Source: three-view drawing plus pictorial views. Frame: mm from the lowest corner of the part. A direction names the side the tool comes from. Give positions to 0.01 mm unless a question says otherwise; leave off trailing zeros. Order: outer loops, then holes, each group sorted by start corner. A loop starts at its lowest first (then second) coordinate and runs counter-clockwise, first axis right, second up.
1) Section C-C, the plane z = 1.55. Return loops of the section in (x, y).
2) Section B-B, the plane y = 17.25. Return loops of the section in (x, z).
3) First-contact query: P1, Ø0.5, axis at y = 13, z = 2, coming from the -X side; P2, Ø1.4, axis at y = 8.5, z = 2, coming from the +X side; P3, Ø0.5, axis at x = 6, z = 2, coming from the -Y side. Flat tips, straight axial feed; report the tip coordinate or a pass-through.
4) Access query for the marked faces 1, 2, 3 and 4. Directions: +Z, -Z, +X, -X, +Y, -Y. A direction counts if a zero-diameter tool reaches every point of the face in a straight line with its end or side. Return the directions, or none.
5) Section A-A, the plane x = 8. Return loops of the section in (y, z), plus the area to 3 significant figures.
6) Draft query along X for the marked faces 5, 6, 7 and 8. Return one class per face: released by +X, released by -X, zero draft, split by the parting line, or undercut.
7) Section D-D, the plane x = 4. Return loops of the section in (y, z), plus the area to 3 significant figures.
8) Material intervals for line 1 (X direction, y = 8, z = 0.65); line 2 (X direction, y = 9, z = 1.4); line 3 (Z direction, x = 1, y = 9.5), sorted ascending.
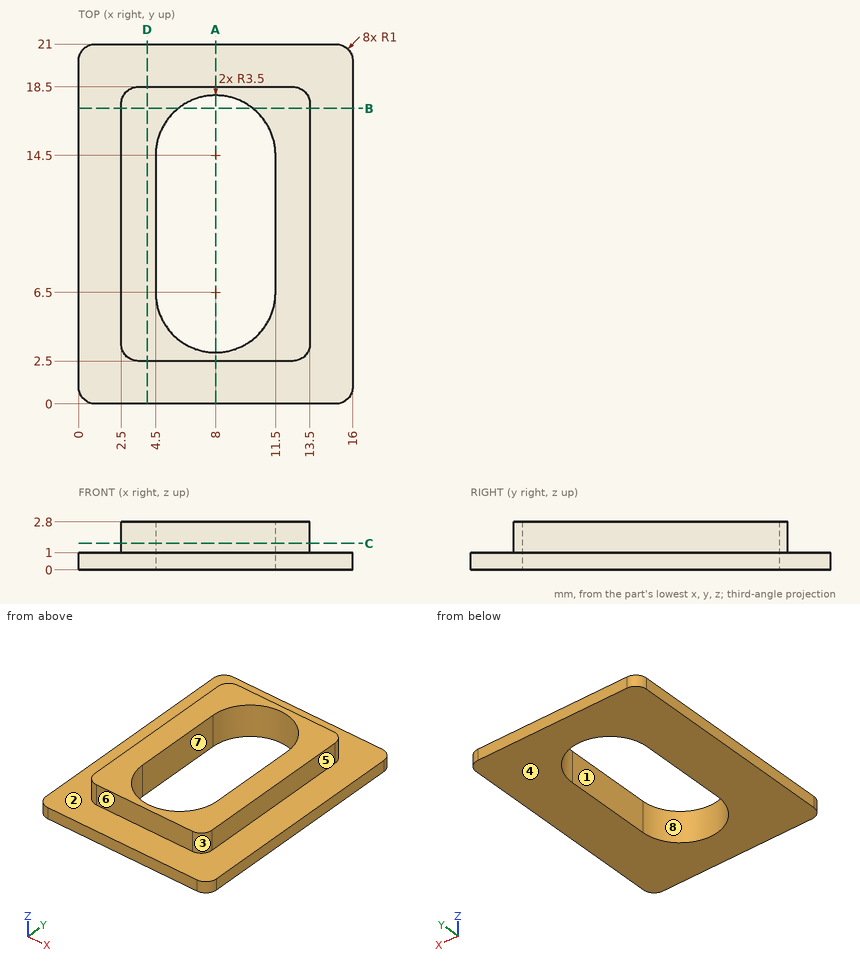
From the geometry:
1. outline: (2.5, 3.5) arc R1 ccw to (3.5, 2.5) - (12.5, 2.5) arc R1 ccw to (13.5, 3.5) - (13.5, 17.5) arc R1 ccw to (12.5, 18.5) - (3.5, 18.5) arc R1 ccw to (2.5, 17.5) - close; hole (4.5, 6.5) arc R3.5 ccw to (11.5, 6.5) - (11.5, 14.5) arc R3.5 ccw to (4.5, 14.5) - close
2. outline: (0, 0) - (5.83, 0) - (5.83, 2.8) - (2.5, 2.8) - (2.5, 1) - (0, 1) - close; (10.17, 0) - (16, 0) - (16, 1) - (13.5, 1) - (13.5, 2.8) - (10.17, 2.8) - close
3. P1: stops at x = 2.5
3. P2: stops at x = 13.5
3. P3: stops at y = 2.5
4. face 1: +Z, -Z
4. face 2: +Z
4. face 3: +Z, +X, -Y
4. face 4: -Z, +X, -X, +Y, -Y
5. outline: (0, 0) - (3, 0) - (3, 2.8) - (2.5, 2.8) - (2.5, 1) - (0, 1) - close; (18, 0) - (21, 0) - (21, 1) - (18.5, 1) - (18.5, 2.8) - (18, 2.8) - close
5. area: 7.80 mm2
6. face 5: released by +X
6. face 6: zero draft
6. face 7: undercut
6. face 8: undercut
7. outline: (0, 0) - (21, 0) - (21, 1) - (18.5, 1) - (18.5, 2.8) - (2.5, 2.8) - (2.5, 1) - (0, 1) - close
7. area: 49.8 mm2
8. line 1: x = 0 to 4.5, 11.5 to 16
8. line 2: x = 2.5 to 4.5, 11.5 to 13.5
8. line 3: z = 0 to 1
